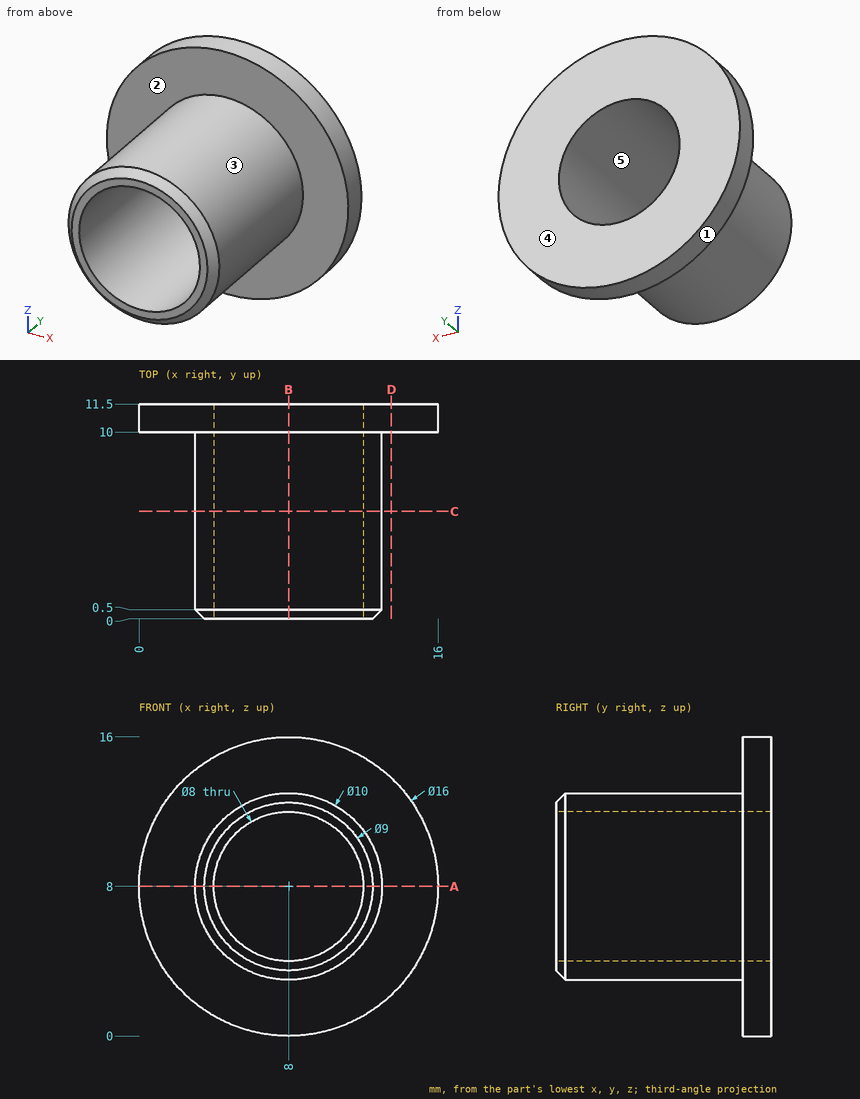
Study the drawing (mm; zero at the part's minimum x, y, z) and answer. A direction names the side the tool comes from. Coordinates: 2 decimals unless noted, no trailing zeros. Write each loop counter-clockwise with the first axis right and the second up, starting at its lowest first coordinate (ties: lowest second). Pieces come first, ordered by that corner, then holes. Notation, with made-up numbers: M 16,81 L 54,81 A16 ccw 54,98 Z; hole C 81,88 d6. An arc over 180 degrees is marked long. Use a Markdown table: item, result. Add a question column.
1. Section D-D (x = 13.5) is taken. Give the vertices of the cut face in (y, z), plus the area to 3 significant figures.
2. For a pull along Z with two mould halves and no side action, classify the marked faces 3, 4 and 5 as +Z half, -Z half, draft (parallel to the pull), parting line (faces both ways), or undercut.
3. Section B-B (x = 8) is taken. Give the vertices of the cut face in (y, z).
4. Which of the six approach directions +Z, -Z, +X, -X, +Y, -Y give full straight-line access (tool end or side, diameter ignored) to the marked faces 1 and 2?
5. Straight lines are drawn through the part: line 1 along Z through (x, y) = (8, 8.25); line 2 along Y through (x, z) = (1, 8.75). For each, find the intervals that lie inside material, in ascending order. Write a range as [from, to].
6. Section A-A (z = 8) is taken. Give the vertices of the cut face in (x, y), plus the area to 4 significant figures.
7. Given P1, Ø8, axis at x = 13, z = 6, coming from the -Y side; P2, Ø1, axis at x = 3.5, z = 13, coming from the -Y side; P3, Ø2, axis at y = 8.5, z = 7.5, coming from the -X side; P4, Ø1, axis at y = 9, z = 11, coming from the -X side, each flat-ended and moving along its own axis, determine where each tip first touches the part or whether it passes through.
8. Section C-C (y = 5.75) is taken. Give the vertices of the cut face in (x, z), plus the area to 3 significant figures.
Data:
| question | item | result |
|---|---|---|
| 1 | outline | M 10,2.19 L 11.5,2.19 L 11.5,13.81 L 10,13.81 Z |
| 1 | area | 17.4 mm2 |
| 2 | face 3 | parting line |
| 2 | face 4 | draft |
| 2 | face 5 | undercut |
| 3 | outline | M 0,3.5 L 0.5,3 L 10,3 L 10,0 L 11.5,0 L 11.5,4 L 0,4 Z; M 0,12 L 11.5,12 L 11.5,16 L 10,16 L 10,13 L 0.5,13 L 0,12.5 Z |
| 4 | face 1 | +Y, -Y |
| 4 | face 2 | -Y |
| 5 | line 1 | z = [3, 4], [12, 13] |
| 5 | line 2 | y = [10, 11.5] |
| 6 | outline | M 0,10 L 3,10 L 3,0.5 L 3.5,0 L 4,0 L 4,11.5 L 0,11.5 Z; M 12,0 L 12.5,0 L 13,0.5 L 13,10 L 16,10 L 16,11.5 L 12,11.5 Z |
| 6 | area | 31.75 mm2 |
| 7 | P1 | stops at y = 0 |
| 7 | P2 | stops at y = 10 |
| 7 | P3 | stops at x = 3 |
| 7 | P4 | stops at x = 3.67 |
| 8 | outline | C 8,8 d10; hole C 8,8 d8 |
| 8 | area | 28.3 mm2 |
